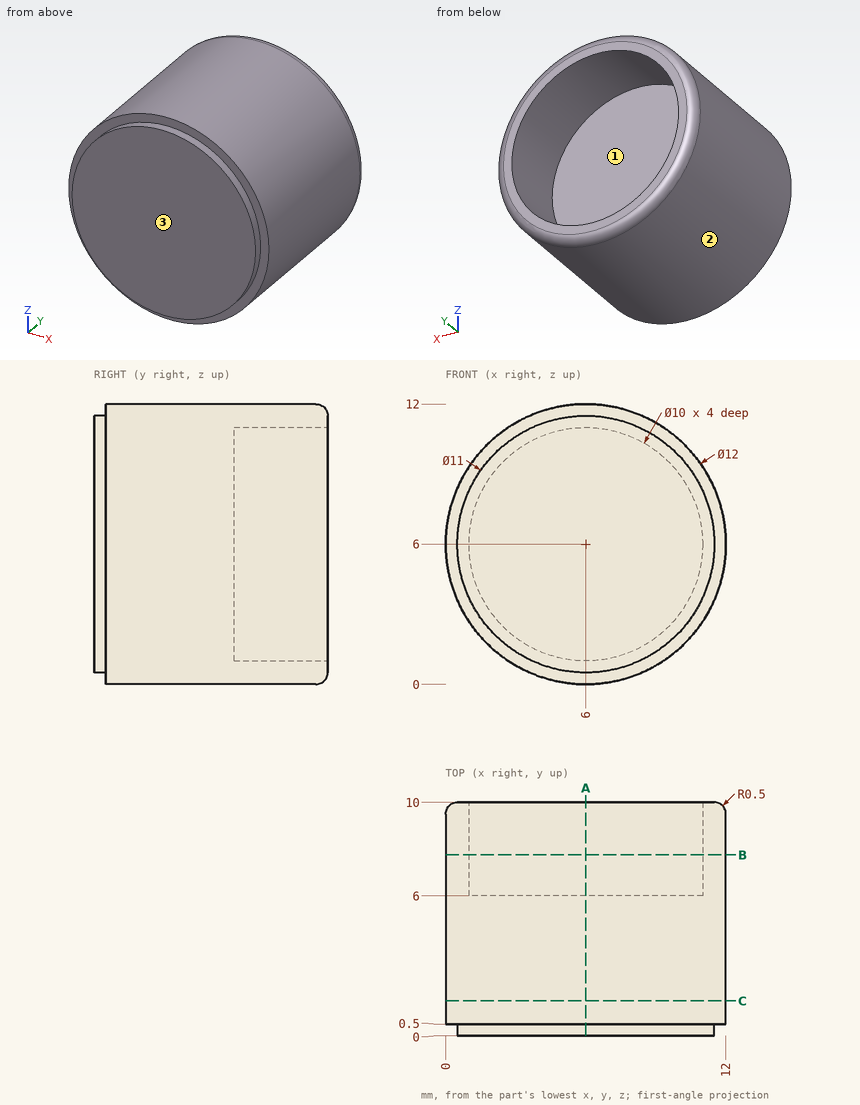
Could you check a few things on this drawing? It's one solid part, dimensions in mm from its lowest x, y, z. Round coordinates to 2 decimals unless told otherwise and drop trailing zeros. Write each loop counter-clockwise with the first axis right and the second up, starting at its lowest first coordinate (ties: lowest second). Pieces come first, ordered by that corner, then holes. Notation, with made-up numbers: (45, 83) -> (87, 83) arc R28 ccw to (87, 108) -> close; hole circle Ø5 at (29, 20). An arc over 180 degrees is marked (long way). One line per item, written item: value.
1) We'd pull the mould along Z, two halves only. Please class the marked faces 1, 2 and 3: released by +Z, released by -Z, zero draft, split by the parting line, or undercut.
Filled sheet:
face 1: undercut
face 2: split by the parting line
face 3: zero draft
2) If I drill on line 1 (Z direction, x = 6, y = 8.9); line 2 (X direction, y = 8.75, z = 3.75); line 3 (Z direction, x = 2.5, y = 8), over which ranges is the centre line in solid material (lowest first)? Write a range as [from, to].
Filled sheet:
line 1: z = [0, 1], [11, 12]
line 2: x = [0.44, 1.53], [10.47, 11.56]
line 3: z = [1.13, 2.43], [9.57, 10.87]
3) Suppose I cut it at C-C on y = 1.5. List the corners of the cut face in (x, z) for me.
Filled sheet:
outline: circle Ø12 at (6, 6)
4) I'm going to push flat-ended pins straight in: pin 1 Ø1 at (y, z) = (1, 3.5) entering from +X; pin 2 Ø3 at (x, y) = (9.5, 4.5) entering from +Z; pin 3 Ø4 at (y, z) = (6.5, 3) entering from -X. Where does each tip first touch, or does it pass through?
Filled sheet:
pin 1: stops at x = 11.66
pin 2: stops at z = 11.66
pin 3: stops at x = 0.08
5) Suppose I cut it at B-B on y = 7.75. List the corners of the cut face in (x, z) for me, plus the area to 3 significant figures.
Filled sheet:
outline: circle Ø12 at (6, 6); hole circle Ø10 at (6, 6)
area: 34.6 mm2
6) Suppose I cut it at A-A on x = 6. List the corners of the cut face in (y, z) for me, plus the area to 3 significant figures.
Filled sheet:
outline: (0, 0.5) -> (0.5, 0.5) -> (0.5, 0) -> (9.5, 0) arc R0.5 ccw to (10, 0.5) -> (10, 1) -> (6, 1) -> (6, 11) -> (10, 11) -> (10, 11.5) arc R0.5 ccw to (9.5, 12) -> (0.5, 12) -> (0.5, 11.5) -> (0, 11.5) -> close
area: 79.4 mm2
